Here's how the part is built. I have some questions about the finished solid (model axes, mm). Coordinates: 2 decimals unless noted, no trailing zeros. Write each loop counter-clockwise with the first axis right and the second up, starting at its lowest first coordinate (ties: lowest second). Pieces come first, ordered by that corner, then holes.
(1) Please list where these lines run through material, in increasing order: probe 1 along X at (y, z) = (0.5, -7); probe 2 along Z at (x, y) = (-11.25, 4.75); probe 3 along Z at (x, y) = (7.75, 2).
(2) For pin 1 Ø2 at (x, y) = (-4, 2.5) entering from +Z; pin 2 Ø1.6 at (y, z) = (5.5, 10.5) entering from +X; pin 3 Ø2 at (x, y) = (10.5, 2.5) entering from -Z, each with a flat end and sliding along its axis, tell me the tip position at first contact or that it passes through.
(3) Imagine slicing it at A-A, the plane z = 7. List the corners of the cut face in (x, y) for me.
(4) Imagine slicing it at D-D, the plane z = -6.25. List the corners of the cut face in (x, y) for me.
(5) Imagine slicing it at B-B, the plane x = 5.5. List the corners of the cut face in (y, z) for me.
(6) Imagine slicing it at C-C, the plane z = -1.5. List the corners of the cut face in (x, y) for me.
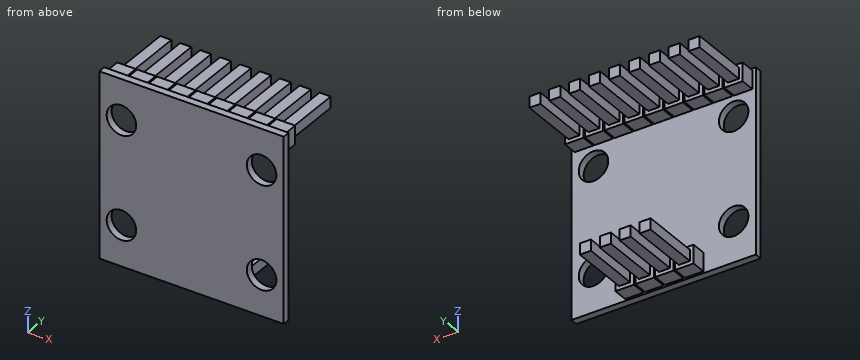
```python
from build123d import *

# Parameters (mm, degrees)
SKETCH_1_W      = 25
SKETCH_1_H      = 25
SKETCH_1_R      = 2
SKETCH_1_W_2    = 2.5
SKETCH_1_H_2    = 2.5
EXTRUDE_1_DEPTH = 1
SKETCH_1_4_W    = 2.5
SKETCH_1_4_H    = 2.5
EXTRUDE_3_DEPTH = 3
SKETCH_3_W      = 1.5
SKETCH_3_H      = 1.5
EXTRUDE_4_DEPTH = 8


with BuildPart() as part:
    # Sketch 1 → Extrude 1 (new body)
    with BuildSketch(Plane(origin=(0, 0, 0), x_dir=(1, 0, 0), z_dir=(0, 1, 0))):
        Rectangle(SKETCH_1_W, SKETCH_1_H)
        with Locations(Location((-9.5, 7, 0), (0, 0, 270))):
            Circle(SKETCH_1_R, mode=Mode.SUBTRACT)
        with Locations(Location((9.5, 7, 0), (0, 0, 270))):
            Circle(SKETCH_1_R, mode=Mode.SUBTRACT)
        with Locations(Location((9.5, -7, 0), (0, 0, 270))):
            Circle(SKETCH_1_R, mode=Mode.SUBTRACT)
        with Locations(Location((-9.5, -7, 0), (0, 0, 270))):
            Circle(SKETCH_1_R, mode=Mode.SUBTRACT)
        with Locations((2.7, -11)):
            Rectangle(SKETCH_1_W_2, SKETCH_1_H_2, mode=Mode.SUBTRACT)
        with Locations((0, -11)):
            Rectangle(SKETCH_1_W_2, SKETCH_1_H_2, mode=Mode.SUBTRACT)
        with Locations((-2.7, -11)):
            Rectangle(SKETCH_1_W_2, SKETCH_1_H_2, mode=Mode.SUBTRACT)
        with Locations((-5.4, -11)):
            Rectangle(SKETCH_1_W_2, SKETCH_1_H_2, mode=Mode.SUBTRACT)
        with Locations((-8.1, -11)):
            Rectangle(SKETCH_1_W_2, SKETCH_1_H_2, mode=Mode.SUBTRACT)
        with Locations((-10.8, -11)):
            Rectangle(SKETCH_1_W_2, SKETCH_1_H_2, mode=Mode.SUBTRACT)
        with Locations((1.25, 11)):
            Rectangle(SKETCH_1_W_2, SKETCH_1_H_2, mode=Mode.SUBTRACT)
        with Locations((-1.45, 11)):
            Rectangle(SKETCH_1_W_2, SKETCH_1_H_2, mode=Mode.SUBTRACT)
        with Locations((3.95, 11)):
            Rectangle(SKETCH_1_W_2, SKETCH_1_H_2, mode=Mode.SUBTRACT)
        with Locations((-4.15, 11)):
            Rectangle(SKETCH_1_W_2, SKETCH_1_H_2, mode=Mode.SUBTRACT)
        with Locations((5.4, -11)):
            Rectangle(SKETCH_1_W_2, SKETCH_1_H_2, mode=Mode.SUBTRACT)
        with Locations((8.1, -11)):
            Rectangle(SKETCH_1_W_2, SKETCH_1_H_2, mode=Mode.SUBTRACT)
        with Locations((10.8, -11)):
            Rectangle(SKETCH_1_W_2, SKETCH_1_H_2, mode=Mode.SUBTRACT)
    extrude(amount=EXTRUDE_1_DEPTH)

    # Sketch 1_4 → Extrude 3 (add)
    with BuildSketch(Plane(origin=(0, 0, 0), x_dir=(1, 0, 0), z_dir=(0, 1, 0))):
        with Locations((2.7, -11)):
            Rectangle(SKETCH_1_4_W, SKETCH_1_4_H)
        with Locations((0, -11)):
            Rectangle(SKETCH_1_4_W, SKETCH_1_4_H)
        with Locations((-2.7, -11)):
            Rectangle(SKETCH_1_4_W, SKETCH_1_4_H)
        with Locations((-5.4, -11)):
            Rectangle(SKETCH_1_4_W, SKETCH_1_4_H)
        with Locations((-8.1, -11)):
            Rectangle(SKETCH_1_4_W, SKETCH_1_4_H)
        with Locations((-10.8, -11)):
            Rectangle(SKETCH_1_4_W, SKETCH_1_4_H)
        with Locations((1.25, 11)):
            Rectangle(SKETCH_1_4_W, SKETCH_1_4_H)
        with Locations((-1.45, 11)):
            Rectangle(SKETCH_1_4_W, SKETCH_1_4_H)
        with Locations((3.95, 11)):
            Rectangle(SKETCH_1_4_W, SKETCH_1_4_H)
        with Locations((-4.15, 11)):
            Rectangle(SKETCH_1_4_W, SKETCH_1_4_H)
        with Locations((5.4, -11)):
            Rectangle(SKETCH_1_4_W, SKETCH_1_4_H)
        with Locations((8.1, -11)):
            Rectangle(SKETCH_1_4_W, SKETCH_1_4_H)
        with Locations((10.8, -11)):
            Rectangle(SKETCH_1_4_W, SKETCH_1_4_H)
    extrude(amount=EXTRUDE_3_DEPTH)

    # Sketch 3 → Extrude 4 (add)
    with BuildSketch(Plane(origin=(0, 3, 0), x_dir=(1, 0, 0), z_dir=(0, 1, 0))):
        with Locations((-4.15, 11)):
            Rectangle(SKETCH_3_W, SKETCH_3_H)
        with Locations((-1.45, 11)):
            Rectangle(SKETCH_3_W, SKETCH_3_H)
        with Locations((1.25, 11)):
            Rectangle(SKETCH_3_W, SKETCH_3_H)
        with Locations((3.95, 11)):
            Rectangle(SKETCH_3_W, SKETCH_3_H)
        with Locations((-8.1, -11)):
            Rectangle(SKETCH_3_W, SKETCH_3_H)
        with Locations((-10.8, -11)):
            Rectangle(SKETCH_3_W, SKETCH_3_H)
        with Locations((-5.4, -11)):
            Rectangle(SKETCH_3_W, SKETCH_3_H)
        with Locations((-2.7, -11)):
            Rectangle(SKETCH_3_W, SKETCH_3_H)
        with Locations((0, -11)):
            Rectangle(SKETCH_3_W, SKETCH_3_H)
        with Locations((2.7, -11)):
            Rectangle(SKETCH_3_W, SKETCH_3_H)
        with Locations((5.4, -11)):
            Rectangle(SKETCH_3_W, SKETCH_3_H)
        with Locations((8.1, -11)):
            Rectangle(SKETCH_3_W, SKETCH_3_H)
        with Locations((10.8, -11)):
            Rectangle(SKETCH_3_W, SKETCH_3_H)
    extrude(amount=EXTRUDE_4_DEPTH)


solid = part.part
```
Recorded:
1. probe 1: x = -12.5 to -11.5, -7.5 to 7.5, 11.5 to 12.5
1. probe 2: z = 10.25 to 11.75
1. probe 3: z = 9.75 to 12.25
2. pin 1: stops at z = 12.25
2. pin 2: stops at x = 11.55
2. pin 3: stops at z = 9.75
3. outline: (-12.5, 0) - (-11.5, 0) - (-11.5, 1) - (-12.5, 1) - close; (-7.5, 0) - (7.5, 0) - (7.5, 1) - (-7.5, 1) - close; (11.5, 0) - (12.5, 0) - (12.5, 1) - (11.5, 1) - close
4. outline: (-12.5, 0) - (-11.35, 0) - (-11.35, 1) - (-12.5, 1) - close; (-7.65, 0) - (7.65, 0) - (7.65, 1) - (-7.65, 1) - close; (11.35, 0) - (12.5, 0) - (12.5, 1) - (11.35, 1) - close
5. outline: (0, -12.5) - (1, -12.5) - (1, 9.75) - (3, 9.75) - (3, 10.25) - (11, 10.25) - (11, 11.75) - (3, 11.75) - (3, 12.25) - (1, 12.25) - (1, 12.5) - (0, 12.5) - close
6. outline: (-12.5, 0) - (12.5, 0) - (12.5, 1) - (-12.5, 1) - close
